Read the model definition and answer for the solid it produces. Units are mm, in the model's axes. Give positions to 0.01 mm unless a question says otherwise; leave off trailing zeros. Loops run counter-clockwise (first coordinate to the right, second up) from the corner with the lowest first, then second, coordinate; pieces in that order, holes last. Notation, with made-up numbers: (30, 47) - (57, 47) arc R20 ccw to (57, 77) - close; hole circle Ø5 at (24, 76). An arc over 180 degrees is marked (long way). Put each result on its own line as item: value. Start each with the question number.
1. A cutting plane is placed at B-B, the plane z = -0.5. Determine the outline of the cut face in (x, y), plus the area to 3 significant figures.
2. For a pull along Z with two mould halves and no side action, classify faces 1 (the flat face through (0, -16, 10)), 2 (the cylindrical face through (0.035, -2.255, -7.861)), 3 (the cylindrical face through (0.14, -8.746, 0.165)), 4 (the flat face through (-10, -16, 0)) as released by +Z, released by -Z, zero draft, split by the parting line, or undercut.
3. A cutting plane is placed at A-A, the plane x = -2. Determine the outline of the cut face in (y, z), plus the area to 3 significant figures.
4. Given pin 1 Ø1.5 at (y, z) = (-8, -1.5) entering from -X; pin 2 Ø3 at (y, z) = (-17, 6) entering from -X; pin 3 Ø5 at (y, z) = (-8, 6.5) entering from +X; pin 4 Ø1 at (y, z) = (-4, 4) entering from +X, each flat-ended and moving along its own axis, determine where each tip first touches the part or whether it passes through.
5. A cutting plane is placed at D-D, the plane y = -7. Determine the outline of the cut face in (x, z), plus the area to 3 significant figures.
6. A cutting plane is placed at C-C, the plane y = -19.5. Determine the outline of the cut face in (x, z).
7. Consider L1, parallel to Y at x = 0.25, z = 0; L2, parallel to Z at x = 4, y = -2.5; L3, parallel to Z at x = 1.25, y = -5. Determine where each line is inside the solid, lowest interval first. Write a range as from..to.
```python
from build123d import *

# Parameters (mm, degrees)
F0_W         = 20
F0_H         = 20
F1_DEPTH     = 25
F2_R         = 3.75
F3_DEPTH     = 25
F4_R         = 7.5
F5_T1_DEPTH  = 36.25
F5_T3_DEPTH  = 5
F5_T6_ANGLE  = 90
F5_T8_ANGLE  = 90
F5_T10_ANGLE = 90
F5_T12_ANGLE = 90


# Not quite as in the source:
# - a fillet or chamfer that OpenCascade refuses, or shapes differently, is made with other operations: its cross-section is extruded or revolved along the edge and cut away or added


with BuildPart() as f1:
    # F0 (on Front) → F1 (new body)
    with BuildSketch(Plane.XZ):
        Rectangle(F0_W, F0_H)
    extrude(amount=F1_DEPTH)

    # F2 (on Right) → F3 (cut, symmetric)
    with BuildSketch(Plane.YZ):
        with Locations((-5, 0)):
            Circle(F2_R)
    extrude(amount=F3_DEPTH, both=True, mode=Mode.SUBTRACT)

    # F4
    f4_edges = [f1.edges().sort_by_distance(p)[0] for p in [
        (0, 0, 10),
        (0, 0, -10),
    ]]
    fillet(f4_edges, radius=F4_R)

    # F5: fillet of radius 7.5 on 8 edges, made by hand

    # F5_s2 → F5_t1 (cut)
    with BuildSketch(Plane.XZ.offset(7.5)):
        with BuildLine():
            ThreePointArc((-10, 2.5), (-7.8033008589, 7.8033008589), (-2.5, 10))
            Line((-2.5, 10), (-10, 10))
            Line((-10, 10), (-10, 2.5))
        make_face()
        with BuildLine():
            ThreePointArc((10, 2.5), (7.8033008589, 7.8033008589), (2.5, 10))
            Line((2.5, 10), (10, 10))
            Line((10, 10), (10, 2.5))
        make_face()
        with BuildLine():
            ThreePointArc((-2.5, -10), (-7.8033008589, -7.8033008589), (-10, -2.5))
            Line((-10, -2.5), (-10, -10))
            Line((-10, -10), (-2.5, -10))
        make_face()
        with BuildLine():
            ThreePointArc((2.5, -10), (7.8033008589, -7.8033008589), (10, -2.5))
            Line((10, -2.5), (10, -10))
            Line((10, -10), (2.5, -10))
        make_face()
    extrude(amount=F5_T1_DEPTH, mode=Mode.SUBTRACT)

    # F5_s4 → F5_t3 (cut)
    with BuildSketch(Plane.XY.offset(-2.5)):
        with BuildLine():
            ThreePointArc((10, -7.5), (7.8033008589, -2.1966991411), (2.5, 0))
            Line((2.5, 0), (10, 0))
            Line((10, 0), (10, -7.5))
        make_face()
        with BuildLine():
            ThreePointArc((-10, -7.5), (-7.8033008589, -2.1966991411), (-2.5, 0))
            Line((-2.5, 0), (-10, 0))
            Line((-10, 0), (-10, -7.5))
        make_face()
    extrude(amount=F5_T3_DEPTH, mode=Mode.SUBTRACT)

    # F5_s5 → F5_t6 (revolve, cut)
    with BuildSketch(Plane.XY.offset(2.5)):
        with BuildLine():
            ThreePointArc((-10, -7.5), (-7.8033008589, -2.1966991411), (-2.5, 0))
            Line((-2.5, 0), (-10, 0))
            Line((-10, 0), (-10, -7.5))
        make_face()
    revolve(axis=Axis((-10, -7.5, 2.5), (1, 0, 0)), revolution_arc=F5_T6_ANGLE, mode=Mode.SUBTRACT)

    # F5_s7 → F5_t8 (revolve, cut)
    with BuildSketch(Plane.XZ.offset(7.5)):
        with BuildLine():
            ThreePointArc((-10, -2.5), (-7.8033008589, -7.8033008589), (-2.5, -10))
            Line((-2.5, -10), (-10, -10))
            Line((-10, -10), (-10, -2.5))
        make_face()
    revolve(axis=Axis((-10, -7.5, -2.5), (1, 0, 0)), revolution_arc=F5_T8_ANGLE, mode=Mode.SUBTRACT)

    # F5_s9 → F5_t10 (revolve, cut)
    with BuildSketch(Plane.XZ.offset(7.5)):
        with BuildLine():
            ThreePointArc((2.5, -10), (7.8033008589, -7.8033008589), (10, -2.5))
            Line((10, -2.5), (10, -10))
            Line((10, -10), (2.5, -10))
        make_face()
    revolve(axis=Axis((10, -7.5, -2.5), (1, 0, 0)), revolution_arc=F5_T10_ANGLE, mode=Mode.SUBTRACT)

    # F5_s11 → F5_t12 (revolve, cut)
    with BuildSketch(Plane.XY.offset(2.5)):
        with BuildLine():
            ThreePointArc((10, -7.5), (7.8033008589, -2.1966991411), (2.5, 0))
            Line((2.5, 0), (10, 0))
            Line((10, 0), (10, -7.5))
        make_face()
    revolve(axis=Axis((10, -7.5, 2.5), (1, 0, 0)), revolution_arc=F5_T12_ANGLE, mode=Mode.SUBTRACT)


solid = f1.part
```
Return value:
1. outline: (-10, -25) - (10, -25) - (10, -8.72) - (-10, -8.72) - close; (-6.7, -1.28) - (6.7, -1.28) arc R7.5 ccw to (2.5, 0) - (-2.5, 0) arc R7.5 ccw to start
1. area: 339 mm2
2. face 1: released by +Z
2. face 2: released by -Z
2. face 3: undercut
2. face 4: zero draft
3. outline: (-25, -10) - (-7.5, -10) arc R7.5 ccw to (0, -2.5) - (0, 2.5) arc R7.5 ccw to (-7.5, 10) - (-25, 10) - close; hole circle Ø7.5 at (-5, 0)
3. area: 432 mm2
4. pin 1: stops at x = -10
4. pin 2: stops at x = -9.73
4. pin 3: stops at x = 9.85
4. pin 4: stops at x = 9.23
5. outline: (-9.95, -3.17) arc R7.48 ccw to (-2.5, -9.98) - (2.5, -9.98) arc R7.48 ccw to (9.95, -3.17) - close; (-9.95, 3.17) - (9.95, 3.17) arc R7.48 ccw to (2.5, 9.98) - (-2.5, 9.98) arc R7.48 ccw to start
5. area: 224 mm2
6. outline: (-10, -2.5) arc R7.5 ccw to (-2.5, -10) - (2.5, -10) arc R7.5 ccw to (10, -2.5) - (10, 2.5) arc R7.5 ccw to (2.5, 10) - (-2.5, 10) arc R7.5 ccw to (-10, 2.5) - close
7. L1: y = -25..-8.75, -1.25..0
7. L2: z = -7.89..-2.8, 2.8..7.89
7. L3: z = -9.57..-3.75, 3.75..9.57
